Here's how the part is built. I have some questions about the finished solid (model axes, mm). A direction names the side the tool comes from. Round coordinates to 2 decimals unless told otherwise and drop trailing zeros. Write each loop counter-clockwise with the first axis right and the second up, starting at its lowest first coordinate (ties: lowest second). Pieces come first, ordered by that corner, then holes. Notation, with made-up numbers: (62, 67) -> (82, 67) arc R9 ccw to (82, 74) -> close; hole circle Ø11 at (30.5, 78). An arc over 180 degrees is marked (long way). Put each result on its own line as item: value. Start each with the question number.
1) Which directions (+Z, -Z, +X, -X, +Y, -Y) give clear straight access to the entire face, cutting with the end or side of a thin tool? Please do faces 4 (the cylindrical face through (25.07, 11.85, 1.52)), 5 (the flat face through (30, 22, -20)).
2) I want a section at D-D, the plane x = 23.5. List the corners of the cut face in (y, z) for me, then the cut area to 3 significant figures.
3) I want a section at A-A, the plane z = -34. List the corners of the cut face in (x, y) for me, then the cut area to 3 significant figures.
4) We'd pull the mould along Z, two halves only. Please class faces 1 (the flat face through (17, 22, 3)), 2 (the cylindrical face through (31.5, 37.5, -21.8)), 3 (the cylindrical face through (24.3, 31, 1.5)): released by +Z, released by -Z, zero draft, split by the parting line, or undercut.
5) If I drill on line 1 along Y through (x, z) = (3.5, 0.65); line 2 along Y through (x, z) = (31.4, -34); line 3 along X through (y, z) = (15.5, -6.5), over which ranges is the centre line in solid material (lowest first)? Write a range as [from, to].
6) I want a section at C-C, the plane y = 6. List the corners of the cut face in (x, z) for me, then the cut area to 3 significant figures.
7) I want a section at B-B, the plane y = 29.75. List the corners of the cut face in (x, z) for me, then the cut area to 3 significant figures.
8) Will these pins go through, and if not, where does the flat tip stop? P1, Ø4.5, axis at x = 3.5, y = 32.5, coming from the -Z side; P2, Ø3, axis at y = 39, z = -21, coming from the +X side; P3, Ø4.5, axis at y = 29.75, z = -34, coming from the -X side; P4, Ø5, axis at x = 14, z = -2, coming from the +Y side.
from build123d import *

# Parameters (mm, degrees)
EXTRUDE_1_DEPTH          = 45
CUT_EXTRUDE_1_REACH      = 86.161
SKETCH_2_R               = 1.7
CUT_EXTRUDE_2_REACH      = 83.939
SKETCH_3_R               = 1.7
SKETCH_3_R_2             = 1.5
CUT_EXTRUDE_3_DEPTH      = 81.777472107
CUT_EXTRUDE_3_DEPTH_BACK = 81.777472107


with BuildPart() as part:
    # 草图1 → 凸台-拉伸1 (new body)
    with BuildSketch(Plane(origin=(0, 0, 0), x_dir=(1, 0, 0), z_dir=(0, 1, 0))):
        Polygon((0, 0), (30, 0), (30, 60), (33, 60), (33, -3), (0, -3), align=None)
    extrude(amount=EXTRUDE_1_DEPTH)

    # 草图2 → 切除-拉伸1 (cut, up to next)
    with BuildSketch(Plane.XY.offset(3), mode=Mode.PRIVATE) as cut_extrude_1_sk1:
        with Locations((3.5, 32.5)):
            Circle(SKETCH_2_R)
    cut_extrude_1_tool1 = extrude(cut_extrude_1_sk1.sketch, amount=-CUT_EXTRUDE_1_REACH, mode=Mode.PRIVATE) & part.part
    # 草图2 → 切除-拉伸1 (cut, up to next)
    with BuildSketch(Plane.XY.offset(3), mode=Mode.PRIVATE) as cut_extrude_1_sk2:
        with Locations((23.5, 32.5)):
            Circle(SKETCH_2_R)
    cut_extrude_1_tool2 = extrude(cut_extrude_1_sk2.sketch, amount=-CUT_EXTRUDE_1_REACH, mode=Mode.PRIVATE) & part.part
    # 草图2 → 切除-拉伸1 (cut, up to next)
    with BuildSketch(Plane.XY.offset(3), mode=Mode.PRIVATE) as cut_extrude_1_sk3:
        with Locations((23.5, 12.5)):
            Circle(SKETCH_2_R)
    cut_extrude_1_tool3 = extrude(cut_extrude_1_sk3.sketch, amount=-CUT_EXTRUDE_1_REACH, mode=Mode.PRIVATE) & part.part
    # 草图2 → 切除-拉伸1 (cut, up to next)
    with BuildSketch(Plane.XY.offset(3), mode=Mode.PRIVATE) as cut_extrude_1_sk4:
        with Locations((3.5, 12.5)):
            Circle(SKETCH_2_R)
    cut_extrude_1_tool4 = extrude(cut_extrude_1_sk4.sketch, amount=-CUT_EXTRUDE_1_REACH, mode=Mode.PRIVATE) & part.part
    add(cut_extrude_1_tool1.solids().sort_by_distance((3.5, 32.5, 3))[0], mode=Mode.SUBTRACT)
    add(cut_extrude_1_tool2.solids().sort_by_distance((23.5, 32.5, 3))[0], mode=Mode.SUBTRACT)
    add(cut_extrude_1_tool3.solids().sort_by_distance((23.5, 12.5, 3))[0], mode=Mode.SUBTRACT)
    add(cut_extrude_1_tool4.solids().sort_by_distance((3.5, 12.5, 3))[0], mode=Mode.SUBTRACT)

    # 草图3 → 切除-拉伸2 (cut, up to next)
    with BuildSketch(Plane(origin=(33, 0, 0), x_dir=(0, 0, -1), z_dir=(1, 0, 0)), mode=Mode.PRIVATE) as cut_extrude_2_sk1:
        with Locations((21, 6)):
            Circle(SKETCH_3_R)
    cut_extrude_2_tool1 = extrude(cut_extrude_2_sk1.sketch, amount=-CUT_EXTRUDE_2_REACH, mode=Mode.PRIVATE) & part.part
    # 草图3 → 切除-拉伸2 (cut, up to next)
    with BuildSketch(Plane(origin=(33, 0, 0), x_dir=(0, 0, -1), z_dir=(1, 0, 0)), mode=Mode.PRIVATE) as cut_extrude_2_sk2:
        with Locations((21, 39)):
            Circle(SKETCH_3_R)
    cut_extrude_2_tool2 = extrude(cut_extrude_2_sk2.sketch, amount=-CUT_EXTRUDE_2_REACH, mode=Mode.PRIVATE) & part.part
    # 草图3 → 切除-拉伸2 (cut, up to next)
    with BuildSketch(Plane(origin=(33, 0, 0), x_dir=(0, 0, -1), z_dir=(1, 0, 0)), mode=Mode.PRIVATE) as cut_extrude_2_sk3:
        with Locations((34, 15.25)):
            Circle(SKETCH_3_R)
    cut_extrude_2_tool3 = extrude(cut_extrude_2_sk3.sketch, amount=-CUT_EXTRUDE_2_REACH, mode=Mode.PRIVATE) & part.part
    # 草图3 → 切除-拉伸2 (cut, up to next)
    with BuildSketch(Plane(origin=(33, 0, 0), x_dir=(0, 0, -1), z_dir=(1, 0, 0)), mode=Mode.PRIVATE) as cut_extrude_2_sk4:
        with Locations((34, 29.75)):
            Circle(SKETCH_3_R)
    cut_extrude_2_tool4 = extrude(cut_extrude_2_sk4.sketch, amount=-CUT_EXTRUDE_2_REACH, mode=Mode.PRIVATE) & part.part
    # 草图3 → 切除-拉伸2 (cut, up to next)
    with BuildSketch(Plane(origin=(33, 0, 0), x_dir=(0, 0, -1), z_dir=(1, 0, 0)), mode=Mode.PRIVATE) as cut_extrude_2_sk5:
        with Locations((26, 39)):
            Circle(SKETCH_3_R_2)
    cut_extrude_2_tool5 = extrude(cut_extrude_2_sk5.sketch, amount=-CUT_EXTRUDE_2_REACH, mode=Mode.PRIVATE) & part.part
    # 草图3 → 切除-拉伸2 (cut, up to next)
    with BuildSketch(Plane(origin=(33, 0, 0), x_dir=(0, 0, -1), z_dir=(1, 0, 0)), mode=Mode.PRIVATE) as cut_extrude_2_sk6:
        with Locations((29.1, 6)):
            Circle(SKETCH_3_R_2)
    cut_extrude_2_tool6 = extrude(cut_extrude_2_sk6.sketch, amount=-CUT_EXTRUDE_2_REACH, mode=Mode.PRIVATE) & part.part
    # 草图3 → 切除-拉伸2 (cut, up to next)
    with BuildSketch(Plane(origin=(33, 0, 0), x_dir=(0, 0, -1), z_dir=(1, 0, 0)), mode=Mode.PRIVATE) as cut_extrude_2_sk7:
        with Locations((29.1, 39)):
            Circle(SKETCH_3_R_2)
    cut_extrude_2_tool7 = extrude(cut_extrude_2_sk7.sketch, amount=-CUT_EXTRUDE_2_REACH, mode=Mode.PRIVATE) & part.part
    # 草图3 → 切除-拉伸2 (cut, up to next)
    with BuildSketch(Plane(origin=(33, 0, 0), x_dir=(0, 0, -1), z_dir=(1, 0, 0)), mode=Mode.PRIVATE) as cut_extrude_2_sk8:
        with Locations((26, 6)):
            Circle(SKETCH_3_R_2)
    cut_extrude_2_tool8 = extrude(cut_extrude_2_sk8.sketch, amount=-CUT_EXTRUDE_2_REACH, mode=Mode.PRIVATE) & part.part
    add(cut_extrude_2_tool1.solids().sort_by_distance((33, 6, -21))[0], mode=Mode.SUBTRACT)
    add(cut_extrude_2_tool2.solids().sort_by_distance((33, 39, -21))[0], mode=Mode.SUBTRACT)
    add(cut_extrude_2_tool3.solids().sort_by_distance((33, 15.25, -34))[0], mode=Mode.SUBTRACT)
    add(cut_extrude_2_tool4.solids().sort_by_distance((33, 29.75, -34))[0], mode=Mode.SUBTRACT)
    add(cut_extrude_2_tool5.solids().sort_by_distance((33, 39, -26))[0], mode=Mode.SUBTRACT)
    add(cut_extrude_2_tool6.solids().sort_by_distance((33, 6, -29.1))[0], mode=Mode.SUBTRACT)
    add(cut_extrude_2_tool7.solids().sort_by_distance((33, 39, -29.1))[0], mode=Mode.SUBTRACT)
    add(cut_extrude_2_tool8.solids().sort_by_distance((33, 6, -26))[0], mode=Mode.SUBTRACT)

    # 草图4 → 切除-拉伸3 (cut, two sides: drawn at the far end of the back side and taken through both)
    with BuildSketch(Plane.ZY.offset(-30).offset(-CUT_EXTRUDE_3_DEPTH_BACK)):
        Polygon((-40, 179.482930557), (-40, 45), (-40, 0), (-40, -134.482930557), (-308.965861114, -134.482930557), (-308.965861114, 179.482930557), align=None)
    extrude(amount=CUT_EXTRUDE_3_DEPTH + CUT_EXTRUDE_3_DEPTH_BACK, mode=Mode.SUBTRACT)


solid = part.part
Findings:
1. face 4: +Z, -Z
1. face 5: -Z, -X, +Y, -Y
2. outline: (0, 0) -> (10.8, 0) -> (10.8, 3) -> (0, 3) -> close; (14.2, 0) -> (30.8, 0) -> (30.8, 3) -> (14.2, 3) -> close; (34.2, 0) -> (45, 0) -> (45, 3) -> (34.2, 3) -> close
2. area: 115 mm2
3. outline: (30, 0) -> (33, 0) -> (33, 13.55) -> (30, 13.55) -> close; (30, 16.95) -> (33, 16.95) -> (33, 28.05) -> (30, 28.05) -> close; (30, 31.45) -> (33, 31.45) -> (33, 45) -> (30, 45) -> close
3. area: 115 mm2
4. face 1: released by +Z
4. face 2: undercut
4. face 3: zero draft
5. line 1: y = [0, 10.8], [14.2, 30.8], [34.2, 45]
5. line 2: y = [0, 13.55], [16.95, 28.05], [31.45, 45]
5. line 3: x = [30, 33]
6. outline: (0, 0) -> (30, 0) -> (30, -19.3) -> (33, -19.3) -> (33, 3) -> (0, 3) -> close; (30, -40) -> (33, -40) -> (33, -30.6) -> (30, -30.6) -> close; (30, -27.6) -> (33, -27.6) -> (33, -27.5) -> (30, -27.5) -> close; (30, -24.5) -> (33, -24.5) -> (33, -22.7) -> (30, -22.7) -> close
6. area: 191 mm2
7. outline: (0, 0) -> (30, 0) -> (30, -32.3) -> (33, -32.3) -> (33, 3) -> (0, 3) -> close; (30, -40) -> (33, -40) -> (33, -35.7) -> (30, -35.7) -> close
7. area: 209 mm2
8. P1: stops at z = 0
8. P2: passes through
8. P3: stops at x = 30
8. P4: stops at y = 45
